Can you work these out from the model? Positions are in its coordinate system, mm. Face numbers are marked on the shaded views. Round coordinates to 2 decimals unless told otherwise and drop trailing zeros. Loops run counter-clockwise (first coordinate to the right, second up) from the corner with the lowest first, then second, coordinate; pieces in that order, holes last.
from build123d import *

# Parameters (mm, degrees)
SKETCH2_W           = 10
SKETCH2_H           = 16
BOSS_EXTRUDE1_DEPTH = 15
CUT_EXTRUDE1_DEPTH  = 23.494443758
FILLET1_R           = 2
SKETCH1_W           = 4
SKETCH1_H           = 1.6
CUT_EXTRUDE3_DEPTH  = 12


with BuildPart() as part:
    # Sketch2 → Boss-Extrude1 (new body)
    with BuildSketch(Plane(origin=(0, 0, 0), x_dir=(1, 0, 0), z_dir=(0, 1, 0))):
        Rectangle(SKETCH2_W, SKETCH2_H)
    extrude(amount=BOSS_EXTRUDE1_DEPTH)

    # Sketch4 → Cut-Extrude1 (cut, through all)
    with BuildSketch(Plane(origin=(0, 0, -8), x_dir=(-1, 0, 0), z_dir=(0, 0, -1))):
        with BuildLine():
            Line((5, 15), (-5, 15))
            ThreePointArc((-5, 15), (0, 14.291616466), (5, 15))
        make_face()
    extrude(amount=-CUT_EXTRUDE1_DEPTH, mode=Mode.SUBTRACT)

    # Fillet1
    fillet1_edges = [part.edges().sort_by_distance(p)[0] for p in [
        (5, 15, 0),
        (-5, 15, 0),
    ]]
    fillet(fillet1_edges, radius=FILLET1_R)

    # Sketch1 → Cut-Extrude3 (cut)
    with BuildSketch(Plane(origin=(0, 0, 0), x_dir=(1, 0, 0), z_dir=(0, 1, 0))):
        Rectangle(SKETCH1_W, SKETCH1_H)
    extrude(amount=CUT_EXTRUDE3_DEPTH, mode=Mode.SUBTRACT)


solid = part.part
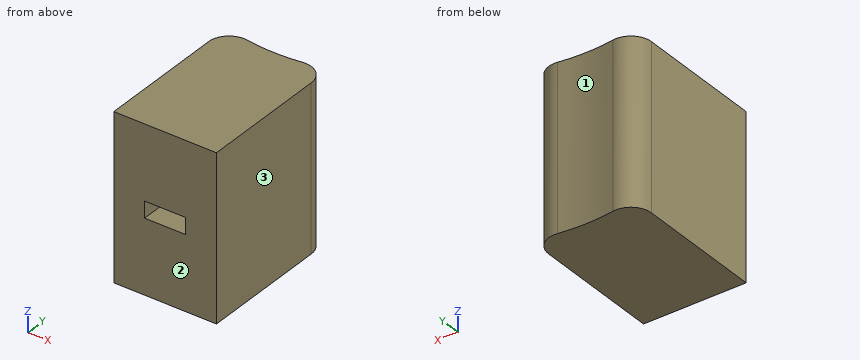
(1) If we mould it in two halves opening along X, with no side actions, what happens to the marked faces 1, 2 and 3? For each: released by +X, released by -X, zero draft, split by the parting line, or undercut.
Worked answers:
face 1: undercut
face 2: zero draft
face 3: released by +X
(2) If we section it at C-C, the plane x = 0.5: List the corners of the cut face in (y, z) for me, then the cut area to 3 significant figures.
Worked answers:
outline: (0, -8) - (14.3, -8) - (14.3, 8) - (0, 8) - (0, 0.8) - (12, 0.8) - (12, -0.8) - (0, -0.8) - close
area: 210 mm2
(3) If we section it at A-A, the plane y = 2.75: List the corners of the cut face in (x, z) for me, then the cut area to 3 significant figures.
Worked answers:
outline: (-5, -8) - (5, -8) - (5, 8) - (-5, 8) - close; hole (-2, -0.8) - (2, -0.8) - (2, 0.8) - (-2, 0.8) - close
area: 154 mm2
(4) If we section it at D-D, the plane z = 0: List the corners of the cut face in (x, y) for me.
Worked answers:
outline: (-5, 0) - (-2, 0) - (-2, 12) - (2, 12) - (2, 0) - (5, 0) - (5, 12.52) arc R2 ccw to (2.7, 14.5) arc R18 cw to (-2.7, 14.5) arc R2 ccw to (-5, 12.52) - close
(5) If we section it at B-B, the plane z = -3.5: List the corners of the cut face in (x, y) for me.
Worked answers:
outline: (-5, 0) - (5, 0) - (5, 12.52) arc R2 ccw to (2.7, 14.5) arc R18 cw to (-2.7, 14.5) arc R2 ccw to (-5, 12.52) - close
(6) If I drill on line 1 (X direction, y = 11.25, z = 0); line 2 (Z direction, x = 1.25, y = 2); line 3 (Y direction, x = 0, z = 5.25), over which ranges is the centre line in solid material (lowest first)?
Worked answers:
line 1: x = -5 to -2, 2 to 5
line 2: z = -8 to -0.8, 0.8 to 8
line 3: y = 0 to 14.29
